Verification items for the finished model (mm, model axes). Face numbers are marked on the shaded views. A direction names the side the tool comes from. Coordinates: 2 decimals unless noted, no trailing zeros. Order: outer loops, then holes, each group sorted by start corner. A loop starts at its lowest first (then second) coordinate and runs counter-clockwise, first axis right, second up.
Q1. Cross-section at C-C, the plane y = 30. Record the boundary of the cut face in (x, z).
Q2. Cross-section at B-B, the plane x = 38. Record the boundary of the cut face in (y, z), and give its area (3 significant figures).
Q3. Cross-section at D-D, the plane x = -13. Record the boundary of the cut face in (y, z), and give its area (3 significant figures).
Q4. Thickness scan on line 1 (Y direction, x = -13, z = 1); line 2 (X direction, y = 14, z = 1); line 3 (X direction, y = 93, z = 5). Record the ranges inside material, lowest first.
Q5. Depth check by flat-ended pin: P1, Ø1.5, axis at y = 71, z = 3.5, coming from the +X side; P2, Ø10, axis at x = -4.5, y = 27, coming from the +Z side; P3, Ø1.4, axis at x = -9.5, z = 1, coming from the -Y side; P4, Ø5, axis at x = 38, y = 14.25, coming from the -Z side. Enter the tip coordinate at first touch or a pass-through.
Q6. Cross-section at A-A, the plane y = 14.25. Record the boundary of the cut face in (x, z).
Q7. Set-up check for the marked faces 1 and 2: record each of +Z, -Z, +X, -X, +Y, -Y from which the full face is reachable in a straight line by a thin tool's end or side.
from build123d import *

# Parameters (mm, degrees)
SKICA1_R                   = 2.25
P_IDAT_VYSUNUT_M10_DEPTH   = 2.8
P_IDAT_VYSUNUT_M10_2_DEPTH = 2.8
P_IDAT_VYSUNUT_M10_3_DEPTH = 2.8
P_IDAT_VYSUNUT_M10_4_DEPTH = 2.8
P_IDAT_VYSUNUT_M11_DEPTH   = 6
SKICA8_R                   = 2.000336871
SKICA8_R_2                 = 2
P_IDAT_VYSUNUT_M12_DEPTH   = 6


with BuildPart() as part:
    # Skica1 → P_idat vysunut_m10 (new body)
    with BuildSketch(Plane.XY):
        with BuildLine():
            Line((-15.25, 81.9), (-4, 81.9))
            Line((-4, 81.9), (-4, 90.4))
            Line((-4, 90.4), (-15.25, 90.4))
            ThreePointArc((-15.25, 90.4), (-16.664213562, 89.814213562), (-17.25, 88.4))
            Line((-17.25, 88.4), (-17.25, 83.9))
            ThreePointArc((-17.25, 83.9), (-16.664213562, 82.485786438), (-15.25, 81.9))
        make_face()
        with Locations((-13, 86.15)):
            Circle(SKICA1_R, mode=Mode.SUBTRACT)
    extrude(amount=P_IDAT_VYSUNUT_M10_DEPTH)



with BuildPart() as body_2:
    # Skica1 → P_idat vysunut_m10 2 (new body)
    with BuildSketch(Plane.XY):
        with BuildLine():
            Line((43.25, 90.4), (29, 90.4))
            Line((29, 90.4), (29, 81.9))
            Line((29, 81.9), (43.25, 81.9))
            ThreePointArc((43.25, 81.9), (45.371320344, 82.778679656), (46.25, 84.9))
            Line((46.25, 84.9), (46.25, 87.4))
            ThreePointArc((46.25, 87.4), (45.371320344, 89.521320344), (43.25, 90.4))
        make_face()
        with Locations((42, 86.15)):
            Circle(SKICA1_R, mode=Mode.SUBTRACT)
    extrude(amount=P_IDAT_VYSUNUT_M10_2_DEPTH)


with BuildPart() as body_3:
    # Skica1 → P_idat vysunut_m10 3 (new body)
    with BuildSketch(Plane.XY):
        with BuildLine():
            Line((29, 18.5), (29, 10))
            Line((29, 10), (39.25, 10))
            ThreePointArc((39.25, 10), (41.371320344, 10.878679656), (42.25, 13))
            Line((42.25, 13), (42.25, 15.5))
            ThreePointArc((42.25, 15.5), (41.371320344, 17.621320344), (39.25, 18.5))
            Line((39.25, 18.5), (29, 18.5))
        make_face()
        with Locations((38, 14.25)):
            Circle(SKICA1_R, mode=Mode.SUBTRACT)
    extrude(amount=P_IDAT_VYSUNUT_M10_3_DEPTH)


with BuildPart() as body_4:
    # Skica1 → P_idat vysunut_m10 4 (new body)
    with BuildSketch(Plane.XY):
        with BuildLine():
            Line((-15.25, 10), (-4, 10))
            Line((-4, 10), (-4, 18.5))
            Line((-4, 18.5), (-15.25, 18.5))
            ThreePointArc((-15.25, 18.5), (-16.664213562, 17.914213562), (-17.25, 16.5))
            Line((-17.25, 16.5), (-17.25, 12))
            ThreePointArc((-17.25, 12), (-16.664213562, 10.585786438), (-15.25, 10))
        make_face()
        with Locations((-13, 14.25)):
            Circle(SKICA1_R, mode=Mode.SUBTRACT)
    extrude(amount=P_IDAT_VYSUNUT_M10_4_DEPTH)


with BuildPart() as part_1:
    add(part.part)

    add(body_2.part)  # P_idat vysunut_m11 merges body 2

    add(body_3.part)  # P_idat vysunut_m11 merges body 3

    add(body_4.part)  # P_idat vysunut_m11 merges body 4
    # Skica1_20 → P_idat vysunut_m11 (add)
    with BuildSketch(Plane.XY):
        with BuildLine():
            Line((25, 103.963290389), (25, 2))
            ThreePointArc((25, 2), (26.963290389, -0.036709611), (29, 1.926580778))
            Line((29, 1.926580778), (29, 106.963290389))
            ThreePointArc((29, 106.963290389), (28.414213562, 108.377503951), (27, 108.963290389))
            Line((27, 108.963290389), (-2, 108.963290389))
            ThreePointArc((-2, 108.963290389), (-3.414213562, 108.377503951), (-4, 106.963290389))
            Line((-4, 106.963290389), (-4, 1.926580778))
            ThreePointArc((-4, 1.926580778), (-1.963290389, -0.036709611), (0, 2))
            Line((0, 2), (0, 104))
            ThreePointArc((0, 104), (0.305319351, 104.683259003), (0.999325975, 104.963290389))
            Line((0.999325975, 104.963290389), (24, 104.963290389))
            ThreePointArc((24, 104.963290389), (24.707106781, 104.67039717), (25, 103.963290389))
        make_face()
    extrude(amount=P_IDAT_VYSUNUT_M11_DEPTH)

    # Skica8 → P_idat vysunut_m12 (add)
    with BuildSketch(Plane.XY.offset(6)):
        with Locations(Location((-2, 1.963290389, 0), (0, 0, 178.948465188))):
            Circle(SKICA8_R)
        with Locations((27, 1.963290389)):
            Circle(SKICA8_R_2)
    extrude(amount=P_IDAT_VYSUNUT_M12_DEPTH)


solid = part_1.part
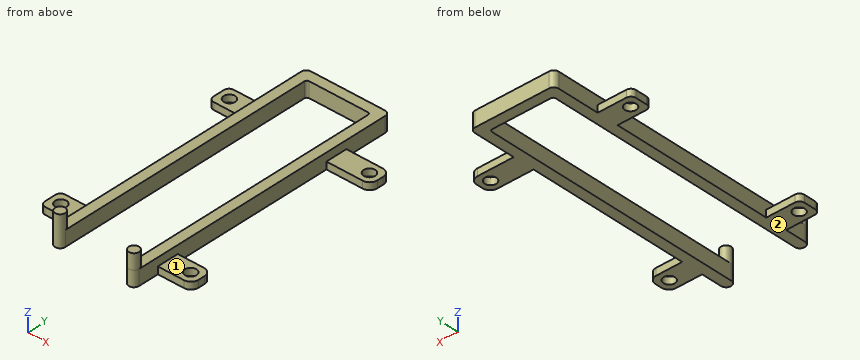
Check values:
1. outline: (-4, 0) - (0, 0) - (0, 6) - (-4, 6) - close; (25, 0) - (29, 0) - (29, 6) - (25, 6) - close
2. outline: (10, 0) - (12, 0) - (12, 2.8) - (10, 2.8) - close; (16.5, 0) - (18.5, 0) - (18.5, 2.8) - (16.5, 2.8) - close; (81.9, 0) - (90.4, 0) - (90.4, 2.8) - (81.9, 2.8) - close
2. area: 35.0 mm2
3. outline: (10, 0) - (12, 0) - (12, 2.8) - (10, 2.8) - close; (16.5, 0) - (18.5, 0) - (18.5, 2.8) - (16.5, 2.8) - close; (81.9, 0) - (83.9, 0) - (83.9, 2.8) - (81.9, 2.8) - close; (88.4, 0) - (90.4, 0) - (90.4, 2.8) - (88.4, 2.8) - close
3. area: 22.4 mm2
4. line 1: y = 10 to 12, 16.5 to 18.5, 81.9 to 83.9, 88.4 to 90.4
4. line 2: x = -17.25 to -15.24, -10.76 to 0, 25 to 35.76, 40.24 to 42.25
4. line 3: x = -4 to 0, 25 to 29
5. P1: stops at x = 29
5. P2: stops at z = 6
5. P3: stops at y = 10
5. P4: stops at z = 0
6. outline: (-17.25, 0) - (-15.25, 0) - (-15.25, 2.8) - (-17.25, 2.8) - close; (-10.75, 0) - (0, 0) - (0, 6) - (-4, 6) - (-4, 2.8) - (-10.75, 2.8) - close; (25, 0) - (35.75, 0) - (35.75, 2.8) - (29, 2.8) - (29, 6) - (25, 6) - close; (40.25, 0) - (42.25, 0) - (42.25, 2.8) - (40.25, 2.8) - close
7. face 1: +Z, +X, +Y, -Y
7. face 2: -Z, +X, -X, +Y, -Y
